Could you check a few things on this model? Use its own coordinates, in mm. A direction names the side the tool comes from. Coordinates: 2 decimals unless noted, no trailing zeros. Order: outer loops, then holes, each group sorted by start corner. A loop starts at its lowest first (then second) coordinate and runs counter-clockwise, first axis right, second up. Notation, with made-up numbers: (84.25, 10.25) -> (130.25, 10.25) arc R19 cw to (130.25, 36.25) -> close; hole circle Ø2 at (23.25, 31.25). An arc over 180 degrees is marked (long way). Put each result on its own line as item: value. Start each with the question number.
Q1. If we section it at B-B (z = 0): Please give me the cut outline in (x, y).
Q2. We'd pull the mould along X, two halves only. Please class faces 4 (the face through (7.778, 3.276, -0.423)), 5 (the face through (10.85, 10.56, -32.72)), 6 (the face through (22, 4, 1)): +X half, -X half, draft (parallel to the pull), parting line (faces both ways), or undercut.
Q3. For faces 1 (the face through (11, 2, 21)), 2 (the face through (12.4, 1.6, 1.4)), 3 (the face through (11, 5, 5)), which set-ups out of +Z, -Z, +X, -X, +Y, -Y let a thin tool reach every point of the face, with its end or its side?
Q4. Please list where these lines run through material, in increasing order: line 1 along Z through (x, y) = (11, 2.5); line 2 along Z through (x, y) = (11, 3.9); line 3 along X through (y, z) = (0.9, 0).
Q5. If we section it at C-C (y = 6.75): Please give me the cut outline in (x, z), and give its area (3 significant figures).
Q6. If we section it at A-A (x = 11): Please give me the cut outline in (y, z).
Q7. Will these pins go through, and if not, where does the flat tip stop? pin 1 (6 mm diameter, centred on x = 17.5, z = 20.5, fed in from +Y); pin 2 (4 mm diameter, centred on x = 14.5, z = 17.5, fed in from +Y); pin 3 (2.5 mm diameter, centred on x = 11, z = 0, fed in from +Y).
Q8. If we section it at D-D (x = 18): Please give me the cut outline in (y, z).
Autodesk Inventor part; units mm, degrees
ref_plane "YZ Plane" through (0, 0, 0) normal (1, 0, 0) x (0, 1, 0)
ref_plane "XZ Plane" through (0, 0, 0) normal (0, 1, 0) x (-1, 0, 0)
ref_plane "XY Plane" through (0, 0, 0) normal (0, 0, 1) x (1, 0, 0)
sketch "Sketch2" plane through (0, 0, 0) normal (1, 0, 0) x (0, 1, 0)
  line L0 (0, 43) -> (0, -43)
  line L1 (0, -43) -> (23.5, -43)
  line L2 (23.5, -43) -> (23.5, -38)
  arc A0 (5, -19.5) -> (23.5, -38) centre (23.5, -19.5) ccw
  line L3 (0, 43) -> (23.5, 43)
  line L4 (23.5, 43) -> (23.5, 38)
  arc A1 (23.5, 38) -> (5, 19.5) centre (23.5, 19.5) ccw
  line L5 (5, 19.5) -> (5, -19.5)
  point P0 (0, 0)
  point P1 (0, 0)
  point P2 (5, 0)
  dimension "d0" = 18.5
  dimension "d1" = 39
  dimension "d2" = 5
  dimension "d3" = 5
extrude "Extrusion1" add sketch "Sketch2" along normal blind 22
sketch "Sketch3" plane through (0, 5, 19.5) normal (0, 1, 0) x (1, 0, 0)
  line L0 (0, 39) -> (0, 0)
  line L1 (0, -23.5) -> (22, -23.5)
  point P0 (0, 19.5)
  point P1 (11, 19.5)
  point P2 (0, 19.5)
  point P3 (11, -23.5)
hole "Hole1" at (11, 5, 0) direction (0, -1, 0) diameter 3.4 end through all counterbore diameter 6.5 counterbore depth 3.4
sketch "Sketch4" plane through (22, 0, 0) normal (1, 0, 0) x (0, 0, -1)
  line L0 (-21, 3.75) -> (-16, 3.75)
  line L1 (-16, 3.75) -> (-16, 1.25)
  line L2 (-16, 1.25) -> (-21, 1.25)
  line L3 (-21, 1.25) -> (-21, 3.75)
  line L4 (16, 3.75) -> (21, 3.75)
  line L5 (21, 3.75) -> (21, 1.25)
  line L6 (21, 1.25) -> (16, 1.25)
  line L7 (16, 1.25) -> (16, 3.75)
  line L8 (-16, 3.75) -> (16, 3.75) construction
  line L9 (-43, 0) -> (43, 0)
  line L10 (-3.25, 5) -> (3.25, 5)
  line L11 (0, 5) -> (0, 0) construction
  point P0 (0, 0)
  point P1 (0, 3.75)
  point P2 (-16, 2.5)
  point P3 (0, 2.5)
  dimension "d13" = 32
  dimension "d14" = 5
  dimension "d15" = 2.5
extrude "Extrusion2" cut sketch "Sketch4" against normal through all
properties part number "CT_Holder"
The answers:
1. outline: (0, 0) -> (9.3, 0) -> (9.3, 1.6) -> (7.75, 1.6) -> (7.75, 5) -> (0, 5) -> close; (12.7, 0) -> (22, 0) -> (22, 5) -> (14.25, 5) -> (14.25, 1.6) -> (12.7, 1.6) -> close
2. face 4: undercut
2. face 5: draft
2. face 6: +X half
3. face 1: +X, -X
3. face 2: +Y
3. face 3: +X, -X, +Y
4. line 1: -43 to -21, -16 to -3.25, 3.25 to 16, 21 to 43
4. line 2: -43 to -3.25, 3.25 to 43
4. line 3: 0 to 9.3, 12.7 to 22
5. outline: (0, -43) -> (22, -43) -> (22, -27.35) -> (0, -27.35) -> close; (0, 27.35) -> (22, 27.35) -> (22, 43) -> (0, 43) -> close
5. area: 688 mm^2
6. outline: (0, -43) -> (23.5, -43) -> (23.5, -38) arc R18.5 cw to (5, -19.5) -> (5, -3.25) -> (1.6, -3.25) -> (1.6, -1.7) -> (0, -1.7) -> close; (0, 1.7) -> (1.6, 1.7) -> (1.6, 3.25) -> (5, 3.25) -> (5, 19.5) arc R18.5 cw to (23.5, 38) -> (23.5, 43) -> (0, 43) -> close; hole (1.25, -21) -> (3.75, -21) -> (3.75, -16) -> (1.25, -16) -> close; hole (1.25, 16) -> (3.75, 16) -> (3.75, 21) -> (1.25, 21) -> close
7. pin 1: y = 5.44
7. pin 2: y = 5
7. pin 3: through
8. outline: (0, -43) -> (23.5, -43) -> (23.5, -38) arc R18.5 cw to (5, -19.5) -> (5, 19.5) arc R18.5 cw to (23.5, 38) -> (23.5, 43) -> (0, 43) -> close; hole (1.25, -21) -> (3.75, -21) -> (3.75, -16) -> (1.25, -16) -> close; hole (1.25, 16) -> (3.75, 16) -> (3.75, 21) -> (1.25, 21) -> close
